Can you work these out from the model? Positions are in its coordinate system, mm. A direction names the side the tool comes from. Coordinates: 2 decimals unless noted, no trailing zeros. Loops run counter-clockwise (first coordinate to the right, second up) from the corner with the lowest first, then second, coordinate; pieces in that order, holes last.
```python
from build123d import *

# Parameters (mm, degrees)
F1_DEPTH = 101.6
F3_DEPTH = 96.52


with BuildPart() as f1:
    # F0 (on Front) → F1 (new body)
    with BuildSketch(Plane.XZ):
        Polygon((48.790029, -5.877001), (20.666308, 44.585982), (-36.017548, 33.432653), (-42.926377, -23.923466), (9.487588, -48.218168), align=None)
    extrude(amount=F1_DEPTH)

    # F2 (on face) → F3 (cut)
    with BuildSketch(Plane.XZ.offset(101.6)):
        Polygon((42.178061, -5.292378), (18.067088, 38.478285), (-31.011986, 29.073266), (-37.23355, -20.510018), (8.000387, -41.749154), align=None)
    extrude(amount=-F3_DEPTH, mode=Mode.SUBTRACT)


solid = f1.part
```
Item 1: We'd pull the mould along Z, two halves only. Please class faces 3 (the face through (-14.933, -54.016, -30.981)), 4 (the face through (2, 0, -1)), 5 (the face through (-7.279, -50.089, 39.087)): +Z half, -Z half, draft (parallel to the pull), parting line (faces both ways), or undercut.
Results are:
face 3: undercut
face 4: draft
face 5: +Z half
Item 2: Suppose I cut it at B-B, the plane z = 18. Please give me the cut outline in (x, y).
Results are:
outline: (-37.88, -101.6) - (-32.4, -101.6) - (-32.4, -5.08) - (29.35, -5.08) - (29.35, -101.6) - (35.48, -101.6) - (35.48, 0) - (-37.88, 0) - close
Item 3: I'm going to push flat-ended pins straight in: P1, Ø12, axis at y = -12.5, z = 34.5, coming from the -X side; P2, Ø1, axis at x = 20, y = -57.5, coming from the +Z side; P3, Ø4, axis at y = -25, z = -15, coming from the -X side. Where does each tip first touch, or does it pass through?
Results are:
P1: stops at x = -36.61
P2: stops at z = 44.55
P3: stops at x = -42.09
Item 4: On a 3-axis mill with a long thin cutter (end or side, diameter ignored), from which of +Z, -Z, +X, -X, +Y, -Y can I reach the whole of each face in a straight line? I mean faces 1 (the face through (-39.424, -50.089, 5.156)), 2 (the face through (2, -5.08, -1)). Say none if no direction works.
Results are:
face 1: +Z, -X, +Y, -Y
face 2: -Y
Item 5: Suppose I cut it at A-A, the plane y = -12. Please give me the cut outline in (x, z), plus the area to 3 significant figures.
Results are:
outline: (-42.93, -23.92) - (9.49, -48.22) - (48.79, -5.88) - (20.67, 44.59) - (-36.02, 33.43) - close; hole (-37.23, -20.51) - (8, -41.75) - (42.18, -5.29) - (18.07, 38.48) - (-31.01, 29.07) - close
area: 1,450 mm2
Item 6: I need wall thicknesses on line 1 along Z through (x, y) = (1, -87.5); line 2 along X through (y, z) = (-57, 11); line 3 along Z through (x, y) = (-26, -28.5). Which ranges of each line are inside material? Lowest first, please.
Results are:
line 1: z = -44.28 to -38.46, 35.21 to 40.72
line 2: x = -38.72 to -33.28, 33.2 to 39.38
line 3: z = -31.77 to -25.78, 30.03 to 35.4
Item 7: Suppose I cut it at C-C, the plane x = -34. Please give me the cut outline in (y, z), plus the area to 3 significant figures.
Results are:
outline: (-101.6, -28.06) - (0, -28.06) - (0, 33.83) - (-101.6, 33.83) - (-101.6, 5.26) - (-5.08, 5.26) - (-5.08, -22.03) - (-101.6, -22.03) - close
area: 3,650 mm2
